CAD build for the part. Positions are in the model's coordinates, mm. A direction names the side the tool comes from. Give positions to 0.01 mm unless a question says otherwise; leave off trailing zeros. Loops run counter-clockwise (first coordinate to the right, second up) from the corner with the lowest first, then second, coordinate; pieces in that order, holes last. Notation, with made-up numbers: M -32,70 L 22,70 A16 cw 22,90 Z; hole C 84,12 d8. An arc over 180 degrees is marked long. One line per question, with ' | ' between items.
```python
from build123d import *

# Parameters (mm, degrees)
EXTRUDE_1_DEPTH     = 3
SKETCH_2_R          = 2.1
CUT_EXTRUDE_1_DEPTH = 3
SKETCH_3_R          = 2.1
CUT_EXTRUDE_2_DEPTH = 129.195163715


with BuildPart() as part:
    # 草图1 → 凸台-拉伸1 (new body)
    with BuildSketch(Plane.XY):
        Polygon((0, 0), (120, 0), (120, 15), (100, 15), (80, 35), (80, 45), (40, 45), (40, 35), (20, 15), (0, 15), align=None)
    extrude(amount=EXTRUDE_1_DEPTH)

    # 草图2 → 切除-拉伸1 (cut)
    with BuildSketch(Plane.XY.offset(3)):
        with Locations((48, 37)):
            Circle(SKETCH_2_R)
        with Locations((72, 37)):
            Circle(SKETCH_2_R)
        with Locations((48, 21)):
            Circle(SKETCH_2_R)
        with Locations((72, 21)):
            Circle(SKETCH_2_R)
        with Locations((8, 8)):
            Circle(SKETCH_2_R)
        with Locations((20, 8)):
            Circle(SKETCH_2_R)
        with Locations((100, 8)):
            Circle(SKETCH_2_R)
        with Locations((112, 8)):
            Circle(SKETCH_2_R)
    extrude(amount=-CUT_EXTRUDE_1_DEPTH, mode=Mode.SUBTRACT)

    # 草图3 → 切除-拉伸2 (cut, through all)
    with BuildSketch(Plane.XY.offset(3)):
        with Locations((32, 8)):
            Circle(SKETCH_3_R)
        with Locations((44, 8)):
            Circle(SKETCH_3_R)
        with Locations((76, 8)):
            Circle(SKETCH_3_R)
        with Locations((88, 8)):
            Circle(SKETCH_3_R)
    extrude(amount=-CUT_EXTRUDE_2_DEPTH, mode=Mode.SUBTRACT)


solid = part.part
```
Item 1: Saw through at D-D on z = 1.1. State how many separate pieces and enclosed holes the cut face has, and give its area (3 significant figures).
Conclusion:
separate pieces: 1 | enclosed holes: 12 | area: 3,230 mm²
Item 2: Drop flat-ended pins along their axis: P1, Ø2.5, axis at x = 76, y = 8, coming from the +Z side; P2, Ø6.5, axis at x = 112, y = 8, coming from the +Z side; P3, Ø1.5, axis at x = 111.5, z = 1, coming from the +Y side. Give the stop position or say it passes through.
Conclusion:
P1: through | P2: z = 3 | P3: y = 15
Item 3: 3-axis set-ups, long thin cutter, end or side, ignore diameter. For faces 4 (the flat face through (0, 8, 1)), 5 (the flat face through (80, 40, 1)), 6 (the flat face through (10, 15, 1)): which of +Z, -Z, +X, -X, +Y, -Y reach the whole face in a straight line?
Conclusion:
face 4: +Z, -Z, -X, +Y, -Y | face 5: +Z, -Z, +X, +Y | face 6: +Z, -Z, -X, +Y
Item 4: Drill centre lines: line 1 along Y through (x, z) = (48, 2.4); line 2 along Y through (x, z) = (44, 1.75); line 3 along Y through (x, z) = (20, 1.65). Where is each one in solid material? Low to high. Write a range as [from, to].
Conclusion:
line 1: [0, 18.9], [23.1, 34.9], [39.1, 45] | line 2: [0, 5.9], [10.1, 45] | line 3: [0, 5.9], [10.1, 15]
Item 5: Mould opens along X. For faces 1 (the cylindrical face through (30.452, 9.419, 1.521)), 2 (the flat face through (30, 25, 1)), 3 (the flat face through (120, 7, 1)) say: pulls with the +X half, pulls with the -X half, needs draft (parallel to the pull), parting line crosses it, or undercut.
Conclusion:
face 1: undercut | face 2: pulls with the -X half | face 3: pulls with the +X half
Item 6: Saw through at A-A on x = 48. Give the cut face in (y, z).
Conclusion:
outline: M 0,0 L 18.9,0 L 18.9,3 L 0,3 Z; M 23.1,0 L 34.9,0 L 34.9,3 L 23.1,3 Z; M 39.1,0 L 45,0 L 45,3 L 39.1,3 Z
Item 7: Saw through at B-B on y = 37. Give the cut face in (x, z), and give its area (3 significant figures).
Conclusion:
outline: M 40,0 L 45.9,0 L 45.9,3 L 40,3 Z; M 50.1,0 L 69.9,0 L 69.9,3 L 50.1,3 Z; M 74.1,0 L 80,0 L 80,3 L 74.1,3 Z | area: 94.8 mm²
Item 8: Saw through at C-C on x = 32. Give the cut face in (y, z), and give its area (3 significant figures).
Conclusion:
outline: M 0,0 L 5.9,0 L 5.9,3 L 0,3 Z; M 10.1,0 L 27,0 L 27,3 L 10.1,3 Z | area: 68.4 mm²
